Part print with two shaded views. Sizes in mm from the minimum x, y, z corner. A direction names the side the tool comes from. Give positions to 0.01 mm unless a question says otherwise; leave off trailing zeros. Order: outer loops, then holes, each group sorted by start corner. A loop starts at its lowest first (then second) coordinate and runs counter-clockwise, first axis right, second up.
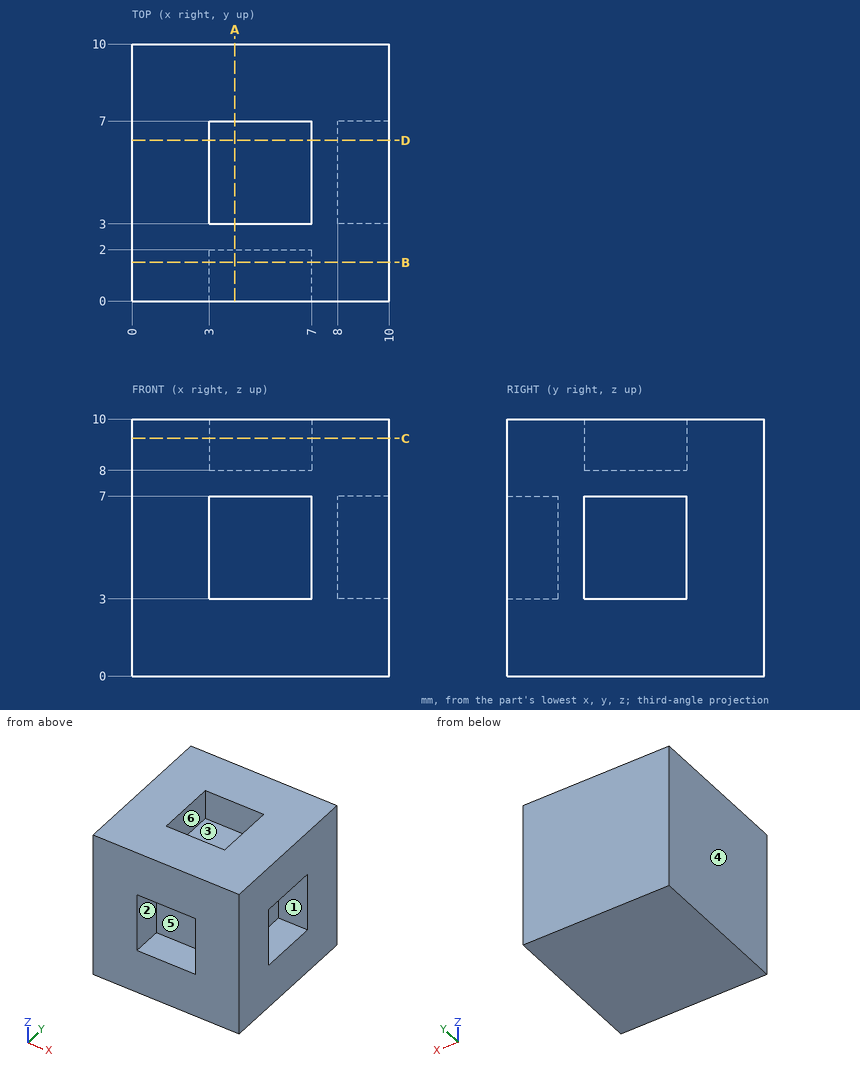
1. Saw through at D-D on y = 6.25. Give the cut face in (x, z).
2. 3-axis set-ups, long thin cutter, end or side, ignore diameter. For the marked faces 1, 2 and 3: which of +Z, -Z, +X, -X, +Y, -Y reach the whole face in a straight line?
3. Saw through at A-A on x = 4. Give the cut face in (y, z).
4. Pin check, flat tips, straight feed: P1, Ø1, axis at y = 6, z = 3.5, coming from the -X side; P2, Ø2, axis at x = 5.5, z = 5.5, coming from the -Y side. Stop position of each tip, or through.
5. Saw through at B-B on y = 1.5. Give the cut face in (x, z).
6. Wall check: line 1 (X direction, y = 5, z = 9); line 2 (Y direction, x = 5.75, z = 4.75). Give the ranges that are in metal, low to high.
7. Mould opens along Y. For the marked faces 4, 5 and 6 say: released by +Y, released by -Y, zero draft, split by the parting line, or undercut.
Reported:
1. outline: (0, 0) - (10, 0) - (10, 3) - (8, 3) - (8, 7) - (10, 7) - (10, 10) - (7, 10) - (7, 8) - (3, 8) - (3, 10) - (0, 10) - close
2. face 1: +X
2. face 2: -Y
2. face 3: +Z
3. outline: (0, 0) - (10, 0) - (10, 10) - (7, 10) - (7, 8) - (3, 8) - (3, 10) - (0, 10) - (0, 7) - (2, 7) - (2, 3) - (0, 3) - close
4. P1: stops at x = 0
4. P2: stops at y = 2
5. outline: (0, 0) - (10, 0) - (10, 10) - (0, 10) - close; hole (3, 3) - (7, 3) - (7, 7) - (3, 7) - close
6. line 1: x = 0 to 3, 7 to 10
6. line 2: y = 2 to 10
7. face 4: zero draft
7. face 5: released by -Y
7. face 6: undercut
